```python
from build123d import *

# Parameters (mm, degrees)
EXTRUDE_1_DEPTH = 44
SKETCH_4_R      = 2.5
EXTRUDE_2_DEPTH = 22


with BuildPart() as part:
    # 草圖1 → 填料-伸長1 (new body)
    with BuildSketch(Plane(origin=(0, 0, 0), x_dir=(1, 0, 0), z_dir=(0, 1, 0))):
        Polygon((-13.5, 0), (-6.5, 0), (-6.5, 5), (-6, 5), (-6, 6), (-6.5, 6), (-6.5, 7), (6.5, 7), (6.5, 6), (6, 6), (6, 5), (6.5, 5), (6.5, 0), (13.5, 0), (13.5, 8), (12.5, 8), (12.5, 9), (13.5, 9), (13.5, 23), (-13.5, 23), (-13.5, 9), (-12.5, 9), (-12.5, 8), (-13.5, 8), align=None)
    extrude(amount=EXTRUDE_1_DEPTH)

    # 除料-掃出1: sweep along a path in 草圖3
    with BuildLine(Plane(origin=(13.5, 0, 0), x_dir=(0, 0, -1), z_dir=(1, 0, 0))) as sweep_1_path:
        Line((23, 34), (18.317914301, 44))
    # 草圖2 → 除料-掃出1 (sweep, cut)
    with BuildSketch(Plane(origin=(0, 0, -23), x_dir=(-1, 0, 0), z_dir=(0, 0, -1))):
        Polygon((-13.5, 44), (-8.5, 44), (-13.5, 34), align=None)
    sweep_1 = sweep(path=sweep_1_path.line, mode=Mode.SUBTRACT)

    # 鏡射1: 除料-掃出1 across plane
    add(sweep_1.mirror(Plane(origin=(0, 0, 0), x_dir=(0, 0, 1), z_dir=(1, 0, 0))), mode=Mode.SUBTRACT)

    # 鏡射2: 除料-掃出1 across plane
    add(sweep_1.mirror(Plane(origin=(0, 22, 0), x_dir=(0, 0, 1), z_dir=(0, -1, 0))), mode=Mode.SUBTRACT)

    # 鏡射2 copy 1: sweep along a path in 鏡射2 copy 1 path
    with BuildLine(Plane(origin=(-13.5, 44, 0), x_dir=(0, 0, -1), z_dir=(-1, 0, 0))) as mirror_2_copy_1_path:
        Line((23, 34), (18.317914301, 44))
    # 鏡射2 copy 1 sketch → 鏡射2 copy 1 (sweep, cut)
    with BuildSketch(Plane(origin=(0, 44, -23), x_dir=(1, 0, 0), z_dir=(0, 0, -1))):
        Polygon((-13.5, 44), (-8.5, 44), (-13.5, 34), align=None)
    sweep(path=mirror_2_copy_1_path.line, mode=Mode.SUBTRACT)

    # 草圖4 → 填料-伸長2 (add, symmetric)
    with BuildSketch(Plane(origin=(0, 0, 0), x_dir=(0, 0, -1), z_dir=(1, 0, 0))):
        with Locations((15, 24)):
            Circle(SKETCH_4_R)
    extrude(amount=EXTRUDE_2_DEPTH, both=True)

    # 草圖5 → 旋轉1 (revolve)
    with BuildSketch(Plane(origin=(22, 0, 0), x_dir=(0, 0, -1), z_dir=(1, 0, 0))):
        with BuildLine():
            Line((15, 28), (15, 20))
            ThreePointArc((15, 20), (19, 24), (15, 28))
        make_face()
    revolve_1 = revolve(axis=Axis((22, 24, -15), (0, 1, 0)))

    # 鏡射3: 旋轉1 across plane
    add(revolve_1.mirror(Plane(origin=(0, 0, 0), x_dir=(0, 0, 1), z_dir=(1, 0, 0))))


solid = part.part
```
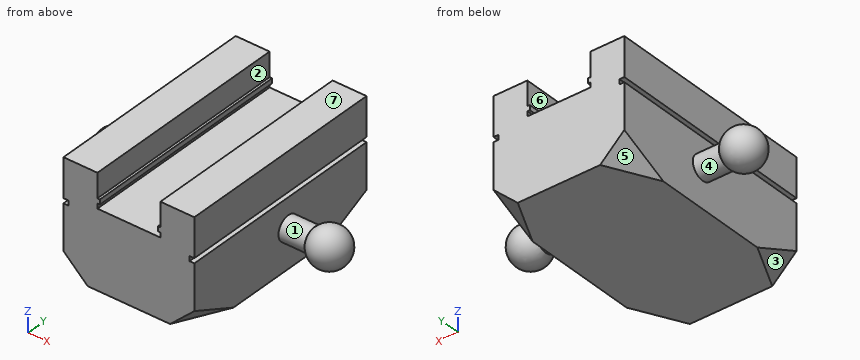
Can you work these out from the model? Positions are in its coordinate system, mm. Face numbers are marked on the shaded views. A direction names the side the tool comes from. Round coordinates to 2 decimals unless told otherwise and drop trailing zeros. Loops run counter-clockwise (first coordinate to the right, second up) from the corner with the lowest first, then second, coordinate; pieces in that order, holes last. Notation, with made-up numbers: (23.5, -12) -> (37.5, -12) arc R9 cw to (37.5, 3) -> close; hole circle Ø7 at (10, -14.5). An arc over 180 degrees is marked (long way). One line per item, written item: value. Start each with the question number.
1. For the marked faces 1, 2 and 3, which set-ups out of +Z, -Z, +X, -X, +Y, -Y let a thin tool reach every point of the face, with its end or its side?
2. If we section it at A-A, the plane z = -3: Write out the boundary of the cut face in (x, y).
3. If we section it at D-D, the plane x = 14.5: Write out the boundary of the cut face in (y, z).
4. For pin 1 (3 mm diameter, centred on y = 7.5, z = -18.5, fed in from +X); pin 2 (0.8 mm diameter, centred on y = 16, z = -5.5, fed in from -X); pin 3 (12 mm diameter, centred on y = 29, z = -8, fed in from +X), each with a flat end and sliding along its axis, tell me the tip position at first contact or that it passes through.
5. If we mould it in two halves opening along X, with no side actions, what happens to the marked faces 4, 5, 6 and 7? For each: pulls with the +X half, pulls with the -X half, needs draft (parallel to the pull), parting line crosses it, or undercut.
6. If we section it at C-C, the plane z = -15: Write out the boundary of the cut face in (x, y).
7. If I drill on probe 1 along X at (y, z) = (39.5, -3); probe 2 along Z at (x, y) = (-1, 42.5); probe 3 along X at (y, z) = (11.5, -17), over which ranges is the centre line in solid material (lowest first)?
Calculated:
1. face 1: none
1. face 2: +Z, +Y, -Y
1. face 3: -Z, -X, -Y
2. outline: (-13.5, 0) -> (-6.5, 0) -> (-6.5, 44) -> (-13.5, 44) -> close; (6.5, 0) -> (13.5, 0) -> (13.5, 44) -> (6.5, 44) -> close
3. outline: circle Ø5 at (24, -15)
4. pin 1: stops at x = 13.5
4. pin 2: stops at x = -13.5
4. pin 3: stops at x = 25.04
5. face 4: undercut
5. face 5: pulls with the -X half
5. face 6: undercut
5. face 7: needs draft
6. outline: (-18.88, 21.5) -> (-13.5, 21.5) -> (-13.5, 0) -> (13.5, 0) -> (13.5, 21.5) -> (18.88, 21.5) arc R4 ccw (long way) to (18.88, 26.5) -> (13.5, 26.5) -> (13.5, 44) -> (-13.5, 44) -> (-13.5, 26.5) -> (-18.88, 26.5) arc R4 ccw (long way) to start
7. probe 1: x = -13.5 to -6.5, 6.5 to 13.5
7. probe 2: z = -23 to -7
7. probe 3: x = -13.5 to 13.5
